from build123d import *

# Parameters (mm, degrees)
F0_W     = 45
F0_H     = 4
F1_DEPTH = 12
F2_R     = 1.6
F3_DEPTH = 4.001
F4_W     = 45
F4_H     = 1
F5_DEPTH = 6.5
F6_R     = 0.5
F7_DEPTH = 7
F8_W     = 10
F8_H     = 9.745784
F9_DEPTH = 6.5


with BuildPart() as f1:
    # F0 (on Top) → F1 (new body)
    with BuildSketch(Plane.XY):
        Rectangle(F0_W, F0_H)
    extrude(amount=F1_DEPTH)

    # F2 (on face) → F3 (cut, through all)
    with BuildSketch(Plane.XZ.offset(2)):
        with Locations((-10, 8.5)):
            Circle(F2_R)
        with Locations((10, 8.5)):
            Circle(F2_R)
    extrude(amount=-F3_DEPTH, mode=Mode.SUBTRACT)

    # F4 (on face) → F5 (cut)
    with BuildSketch(Plane(origin=(0, 0, 0), x_dir=(1, 0, 0), z_dir=(0, 0, -1))):
        with Locations((0, -1.5)):
            Rectangle(F4_W, F4_H)
    extrude(amount=-F5_DEPTH, mode=Mode.SUBTRACT)

    # F6 (on face) → F7 (join)
    with BuildSketch(Plane(origin=(0, 0, 0), x_dir=(1, 0, 0), z_dir=(0, 0, -1))):
        with Locations((22, -1)):
            Circle(F6_R)
        with Locations((20, -1)):
            Circle(F6_R)
        with Locations((18, -1)):
            Circle(F6_R)
        with Locations((16, -1)):
            Circle(F6_R)
        with Locations((14, -1)):
            Circle(F6_R)
        with Locations((12, -1)):
            Circle(F6_R)
        with Locations((10, -1)):
            Circle(F6_R)
        with Locations((8, -1)):
            Circle(F6_R)
        with Locations((6, -1)):
            Circle(F6_R)
        with Locations((4, -1)):
            Circle(F6_R)
        with Locations((2, -1)):
            Circle(F6_R)
        with Locations((0, -1)):
            Circle(F6_R)
        with Locations((-2, -1)):
            Circle(F6_R)
        with Locations((-4, -1)):
            Circle(F6_R)
        with Locations((-6, -1)):
            Circle(F6_R)
        with Locations((-8, -1)):
            Circle(F6_R)
        with Locations((-10, -1)):
            Circle(F6_R)
        with Locations((-12, -1)):
            Circle(F6_R)
        with Locations((-14, -1)):
            Circle(F6_R)
        with Locations((-16, -1)):
            Circle(F6_R)
        with Locations((-18, -1)):
            Circle(F6_R)
        with Locations((-20, -1)):
            Circle(F6_R)
        with Locations((-22, -1)):
            Circle(F6_R)
    extrude(amount=-F7_DEPTH)

    # F8 (on face) → F9 (cut)
    with BuildSketch(Plane(origin=(0, 0, 0), x_dir=(1, 0, 0), z_dir=(0, 0, -1))):
        Rectangle(F8_W, F8_H)
    extrude(amount=-F9_DEPTH, mode=Mode.SUBTRACT)


solid = f1.part
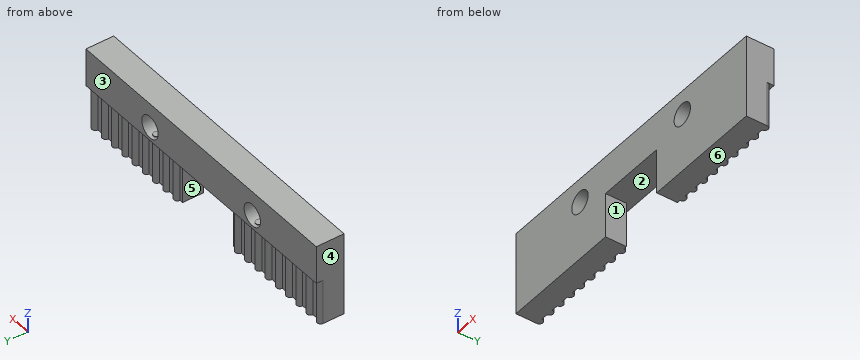
Model file for the job. Use its own axes, mm. Face numbers are marked on the shaded views. A direction names the side the tool comes from. Coordinates: 2 decimals unless noted, no trailing zeros. Loops run counter-clockwise (first coordinate to the right, second up) from the corner with the lowest first, then second, coordinate; pieces in that order, holes last. Notation, with made-up numbers: (-23, 1.25) -> (17, 1.25) arc R32 ccw to (17, 30.25) -> close; hole circle Ø11 at (-24.5, -35.75). An arc over 180 degrees is marked (long way). Use one line per item in the form item = value. Start each with the question number.
(1) Flat gauge pins, fed straight in: pin 1 (0.5 mm diameter, centred on x = -21, z = 2.5, fed in from +Y); pin 2 (1.5 mm diameter, centred on x = 15, y = 0, fed in from -Z). Where does each tip first touch, or does it go through?
(2) Cut at B-B on y = -0.2. Give the cut face in (x, z).
(3) Cut at A-A on x = -10. Give the cut face in (y, z), and give its area (4 significant figures).
(4) Tool access for the marked faces 1, 2 and 3: list every direction of +Z, -Z, +X, -X, +Y, -Y with a clear straight run to the whole face (end or side of a thin tool).
(5) Probe probe 1 along Z at (x, y) = (10, 0.65); probe 2 along Z at (x, y) = (-10, 0.1); probe 3 along X at (y, z) = (0.95, 8.75). List the from-to ranges inside material, lowest first. Write a range as from..to.
(6) Pull direction X, two halves, no side cores. Call the marked faces 4, 5 and 6: pulls with the +X half, pulls with the -X half, needs draft (parallel to the pull), parting line crosses it, or undercut.
Values:
q1.pin_1 = 1
q1.pin_2 = 0
q2.outline = (-22.5, 0) -> (-5, 0) -> (-5, 6.5) -> (5, 6.5) -> (5, 0) -> (22.5, 0) -> (22.5, 12) -> (-22.5, 12) -> close; hole circle Ø3.2 at (-10, 8.5); hole circle Ø3.2 at (10, 8.5)
q3.outline = (-2, 0) -> (1.5, 0) -> (1.5, 6.5) -> (2, 6.5) -> (2, 6.9) -> (1.5, 6.9) -> (1.5, 7) -> (0.5, 7) -> (0.5, 6.9) -> (-2, 6.9) -> close; (-2, 10.1) -> (2, 10.1) -> (2, 12) -> (-2, 12) -> close
q3.area = 32.05 mm2
q4.face_1 = -Z, +Y, -Y
q4.face_2 = -Z, +Y
q4.face_3 = +Z, -Z, +X, -X, +Y
q5.probe_1 = 0..7, 10.1..12
q5.probe_2 = 0..6.9, 10.1..12
q5.probe_3 = -22.5..-11.58, -8.42..8.42, 11.58..22.5
q6.face_4 = pulls with the -X half
q6.face_5 = undercut
q6.face_6 = needs draft
